Can you work these out from the drawing? Everything is in mm from the part's minimum corner. Round coordinates to 2 decimals unless told otherwise and drop trailing zeros. Loops run counter-clockwise (first coordinate to the right, second up) from the corner with the lowest first, then second, coordinate; pieces in that order, holes last. Notation, with made-up numbers: (-30, -18) -> (-6, -18) arc R15 ccw to (-6, 1) -> close; hole circle Ø9 at (-38.75, 29). An arc over 180 degrees is marked (long way). Use CSV: the item, a comma, the result in double quotes. Start each with the question number.
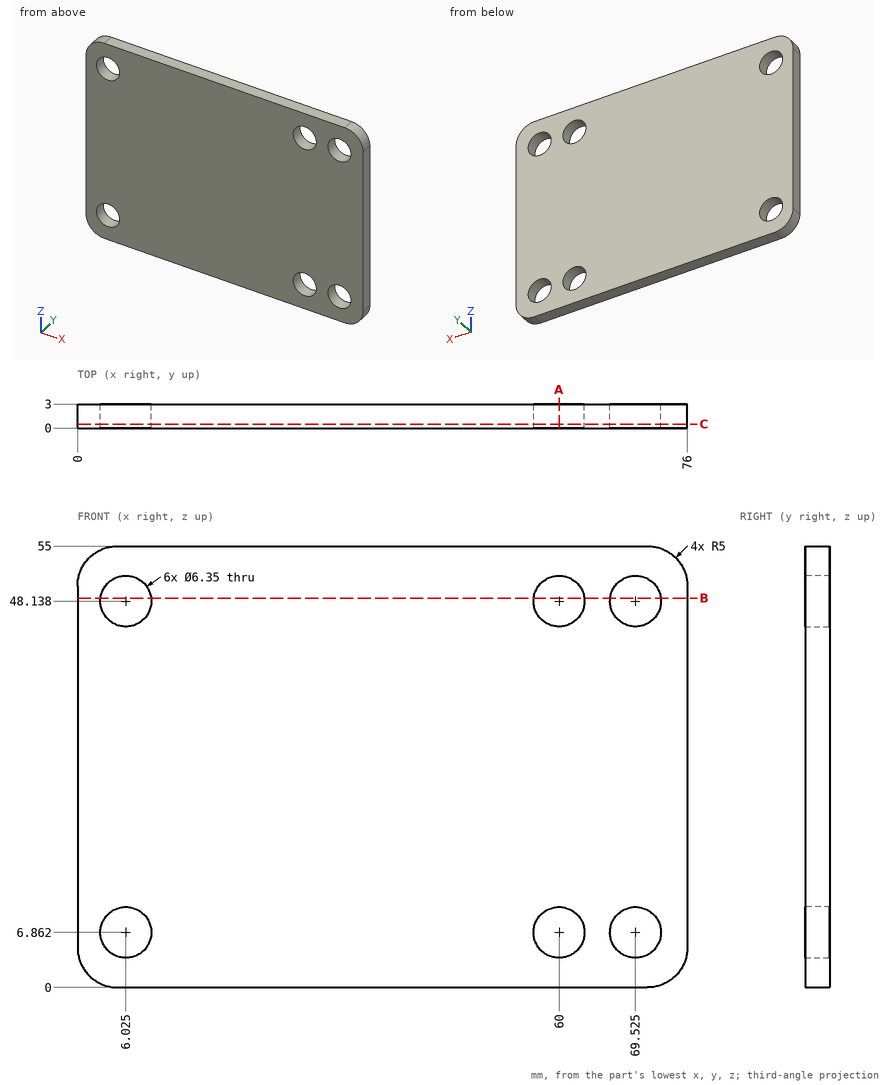
1. If I drill on L1, parallel to Z at x = 6.5, y = 1.2; L2, parallel to X at y = 2.5, z = 45.5 (1 decimal); L3, parallel to Z at x = 68.5, y = 1.4, over which ranges is the centre line in solid material (lowest first)?
2. Suppose I cut it at C-C (y = 0.5). State how many separate pieces and enclosed holes the cut face has, then the cut area to 3 significant figures.
3. Suppose I cut it at B-B (z = 48.5). List the corners of the cut face in (x, y) for me (1 decimal), then the cut area to 3 significant figures.
4. Suppose I cut it at A-A (x = 60). List the corners of the cut face in (y, z) for me.
Geometry check:
1,L1,"z = 0 to 3.72, 10 to 45, 51.28 to 55"
1,L2,"x = 0 to 4.3, 7.8 to 58.2, 61.8 to 67.8, 71.3 to 76"
1,L3,"z = 0 to 3.86, 9.87 to 45.13, 51.14 to 55"
2,separate pieces,"1"
2,enclosed holes,"6"
2,area,"3,970 mm²"
3,outline,"(0, 0) -> (2.9, 0) -> (2.9, 3) -> (0, 3) -> close; (9.2, 0) -> (56.8, 0) -> (56.8, 3) -> (9.2, 3) -> close; (63.2, 0) -> (66.4, 0) -> (66.4, 3) -> (63.2, 3) -> close; (72.7, 0) -> (76, 0) -> (76, 3) -> (72.7, 3) -> close"
3,area,"171 mm²"
4,outline,"(0, 0) -> (3, 0) -> (3, 3.69) -> (0, 3.69) -> close; (0, 10.04) -> (3, 10.04) -> (3, 44.96) -> (0, 44.96) -> close; (0, 51.31) -> (3, 51.31) -> (3, 55) -> (0, 55) -> close"
